Geometry check sheet. Reference: the model listing, model coordinates, mm. Round coordinates to 2 decimals unless told otherwise and drop trailing zeros. Write each loop counter-clockwise with the first axis right and the second up, starting at its lowest first coordinate (ties: lowest second). Pieces come first, ordered by that corner, then holes. Notation, with made-up numbers: M 1,5.25 L 55,5.25 A15 cw 55,30.25 Z; hole C 40,69.25 d3. An arc over 180 degrees is marked long. Use a Markdown table: item, result.
```python
from build123d import *

# Parameters (mm, degrees)
SKETCH1_W               = 250
SKETCH1_H               = 45.72
BOSS_EXTRUDE1_DEPTH     = 3
CUT_EXTRUDE1_DEPTH      = 128.108534725
CUT_EXTRUDE1_DEPTH_BACK = 128.108534725
SKETCH2_W               = 12
SKETCH2_H               = 10


with BuildPart() as part:
    # Sketch1 → Boss-Extrude1 (new body)
    with BuildSketch(Plane(origin=(0, 0, 0), x_dir=(1, 0, 0), z_dir=(0, 1, 0))):
        Rectangle(SKETCH1_W, SKETCH1_H)
    extrude(amount=BOSS_EXTRUDE1_DEPTH)

    # Sketch2 → Cut-Extrude1 (cut, two sides: drawn at the far end of the back side and taken through both)
    with BuildSketch(Plane(origin=(0, 0, 0), x_dir=(1, 0, 0), z_dir=(0, 1, 0)).offset(-CUT_EXTRUDE1_DEPTH_BACK)):
        with Locations((-25, 0)):
            Rectangle(SKETCH2_W, SKETCH2_H)
        with Locations((10, 0)):
            Rectangle(SKETCH2_W, SKETCH2_H)
        with Locations((45, 0)):
            Rectangle(SKETCH2_W, SKETCH2_H)
    extrude(amount=CUT_EXTRUDE1_DEPTH + CUT_EXTRUDE1_DEPTH_BACK, mode=Mode.SUBTRACT)


solid = part.part
```
Item 1: Cross-section at A-A, the plane y = 0.75. Record the cut outline in (x, z), and give its area (3 significant figures).
Outcome:
| item | result |
|---|---|
| outline | M -125,-22.86 L 125,-22.86 L 125,22.86 L -125,22.86 Z; hole M -31,-5 L -19,-5 L -19,5 L -31,5 Z; hole M 4,-5 L 16,-5 L 16,5 L 4,5 Z; hole M 39,-5 L 51,-5 L 51,5 L 39,5 Z |
| area | 11,100 mm2 |
Item 2: Cross-section at B-B, the plane z = -1. Record the cut outline in (x, y).
Outcome:
| item | result |
|---|---|
| outline | M -125,0 L -31,0 L -31,3 L -125,3 Z; M -19,0 L 4,0 L 4,3 L -19,3 Z; M 16,0 L 39,0 L 39,3 L 16,3 Z; M 51,0 L 125,0 L 125,3 L 51,3 Z |
Item 3: Go/stop test with a flat-tipped pin: pin 1 (12 mm diameter, centred on x = -57.5, z = 10, fed in from -Y). Record where the tip stops, or that it passes through.
Outcome:
| item | result |
|---|---|
| pin 1 | stops at y = 0 |
Item 4: Cross-section at C-C, the plane x = 46. Record the cut outline in (y, z).
Outcome:
| item | result |
|---|---|
| outline | M 0,-22.86 L 3,-22.86 L 3,-5 L 0,-5 Z; M 0,5 L 3,5 L 3,22.86 L 0,22.86 Z |
Item 5: Material ranges on line 1 along X through (y, z) = (2.2, -3.5); line 2 along Z through (x, y) = (42.5, 1.95), recorded low to high. Write a range as from..to.
Outcome:
| item | result |
|---|---|
| line 1 | x = -125..-31, -19..4, 16..39, 51..125 |
| line 2 | z = -22.86..-5, 5..22.86 |
